from build123d import *

# Parameters (mm, degrees)
F1_DEPTH = 252.4125
F4_R     = 101.6
F5_DEPTH = 9.525
F6_W     = 19.05
F6_H     = 85.852
F7_DEPTH = 6.35


with BuildPart() as f1:
    # F0 (on Front) → F1 (new body)
    with BuildSketch(Plane.XZ):
        Polygon((9.525, 52.451), (-9.525, 52.451), (-9.525, -33.401), (0, -33.401), (0, -46.101), (-9.525, -46.101), (-9.525, -52.451), (9.525, -52.451), align=None)
    extrude(amount=F1_DEPTH)

    # F3: F1 across plane


with BuildPart() as f1_1:
    add(f1.part)
    add(f1.part.mirror(Plane.XZ))

    # F4 (on Top) → F5 (cut, symmetric)
    with BuildSketch(Plane.XY):
        with Locations((101.6, 0)):
            Circle(F4_R)
    extrude(amount=F5_DEPTH, both=True, mode=Mode.SUBTRACT)

    # F6 (on face) → F7 (cut)
    with BuildSketch(Plane(origin=(-9.525, 0, 0), x_dir=(0, -1, 0), z_dir=(-1, 0, 0))):
        with Locations((-19.05, 9.525)):
            Rectangle(F6_W, F6_H)
        with Locations((19.05, 9.525)):
            Rectangle(F6_W, F6_H)
    extrude(amount=-F7_DEPTH, mode=Mode.SUBTRACT)


solid = f1_1.part
The listing builds one solid part. Answer for the finished solid, in the listing's coordinates (mm). A direction names the side the tool comes from. Coordinates: 2 decimals unless noted, no trailing zeros. Write each loop counter-clockwise with the first axis right and the second up, starting at its lowest first coordinate (ties: lowest second). Pieces come first, ordered by that corner, then holes. Notation, with made-up numbers: (-39.75, 45.25) - (-35.75, 45.25) arc R17 cw to (-35.75, 49.25) - close; hole circle Ø7 at (57.5, -25). An arc over 180 degrees is marked (long way). Return JSON: item names as keys, results as strings.
1. Which of the six approach directions +Z, -Z, +X, -X, +Y, -Y give full straight-line access (tool end or side, diameter ignored) to faces 1 (the face through (0, 252.412, 1)), 2 (the face through (-3.175, -19, 10)), 3 (the face through (0, -4, -40)), 4 (the face through (0, 0.6, 0.1))?
Final values:
{"face 1": "+Z, -Z, +X, -X, +Y", "face 2": "+Z, -X", "face 3": "-X, +Y, -Y", "face 4": "+X"}
2. Each of these flat-tipped pins is pushed along its axis until it touches: pin 1 Ø4 at (y, z) = (7, -41) entering from -X; pin 2 Ø9.5 at (y, z) = (18, 17) entering from -X (3 decimals). Where does it stop, or does it pass through?
Final values:
{"pin 1": "x = 0", "pin 2": "x = -3.175"}
3. The part is cut by section C-C on z = -25. Determine the outline of the cut face in (x, y) (1 decimal).
Final values:
{"outline": "(-9.5, -252.4) - (9.5, -252.4) - (9.5, 252.4) - (-9.5, 252.4) - (-9.5, 28.6) - (-3.2, 28.6) - (-3.2, 9.5) - (-9.5, 9.5) - (-9.5, -9.5) - (-3.2, -9.5) - (-3.2, -28.6) - (-9.5, -28.6) - close"}
4. The part is cut by section A-A on x = 6.25. Determine the outline of the cut face in (y, z) (1 decimal), then the cut area to 3 significant figures.
Final values:
{"outline": "(-252.4, -52.5) - (252.4, -52.5) - (252.4, 52.5) - (-252.4, 52.5) - close; hole (-35.1, -9.5) - (35.1, -9.5) - (35.1, 9.5) - (-35.1, 9.5) - close", "area": "51,600 mm^2"}
5. The part is cut by section B-B on y = 91.5. Determine the outline of the cut face in (x, z) (3 decimals), then the cut area to 3 significant figures.
Final values:
{"outline": "(-9.525, -52.451) - (9.525, -52.451) - (9.525, 52.451) - (-9.525, 52.451) - (-9.525, -33.401) - (0, -33.401) - (0, -46.101) - (-9.525, -46.101) - close", "area": "1,880 mm^2"}
6. For a pull along Z with two mould halves and no side action, classify faces 5 (the face through (0, -4, 52.451)), 6 (the face through (6, 1, -9.525)), 7 (the face through (-9.525, 139, 10)) as +Z half, -Z half, draft (parallel to the pull), parting line (faces both ways), or undercut.
Final values:
{"face 5": "+Z half", "face 6": "undercut", "face 7": "draft"}
7. Consider line 1 along Y through (x, z) = (-7.5, -24) (1 decimal); line 2 along Z through (x, y) = (-5, -81); line 3 along X through (y, z) = (28, -16) (3 decimals). Determine where each line is inside the solid, lowest interval first.
Final values:
{"line 1": "-252.4 to -28.6, -9.5 to 9.5, 28.6 to 252.4", "line 2": "-52.45 to -46.1, -33.4 to 52.45", "line 3": "-3.175 to 9.525"}
8. The part is cut by section D-D on y = 20.5. Determine the outline of the cut face in (x, z) (3 decimals).
Final values:
{"outline": "(-9.525, -52.451) - (9.525, -52.451) - (9.525, -9.525) - (2.09, -9.525) - (2.09, 9.525) - (9.525, 9.525) - (9.525, 52.451) - (-3.175, 52.451) - (-3.175, -33.401) - (0, -33.401) - (0, -46.101) - (-9.525, -46.101) - close"}
